Part model, mm, in its own coordinate system. Coordinates: 2 decimals unless noted, no trailing zeros. Loops run counter-clockwise (first coordinate to the right, second up) from the corner with the lowest first, then second, coordinate; pieces in that order, holes last. Notation, with made-up numbers: (-25.5, 3.25) - (-4.5, 3.25) arc R12 cw to (-4.5, 14.25) - close; hole circle Ø4 at (-8.75, 41.5). An arc over 180 degrees is marked (long way). Use a Markdown table: item, result. Add a question column.
1. Band-saw the part on A-A, the plane y = 133.5. Give the cut face in (x, z).
2. Wall check: probe 1 along Y at (x, z) = (48.8, 3.4); probe 2 along X at (y, z) = (133.5, 3.25); probe 3 along X at (y, z) = (41.5, 1.8). Give the ranges that are in metal, low to high. Write a range as [from, to].
3. Band-saw the part on C-C, the plane x = 28.8. Give the cut face in (y, z), plus the area to 3 significant figures.
4. Band-saw the part on B-B, the plane z = 3.85. Count the separate pieces of the cut face and the enclosed holes in it, plus the area to 3 significant figures.
5. Drop flat-ended pins along their axis: pin 1 (2 mm diameter, centred on y = 82, z = 2.5, fed in from +X); pin 2 (1.5 mm diameter, centred on y = 3.5, z = 1.5, fed in from +X); pin 3 (1.5 mm diameter, centred on x = 3.5, z = 1.5, fed in from +Y). Give the stop position or say it passes through.
6. Band-saw the part on D-D, the plane y = 75.5. Give the cut face in (x, z), plus the area to 3 significant figures.
from build123d import *

# Parameters (mm, degrees)
SKETCH_1_W          = 77.6
SKETCH_1_H          = 137
EXTRUDE_1_DEPTH     = 5
SKETCH_3_W          = 18.8
SKETCH_3_H          = 7.5
SKETCH_3_W_2        = 5
SKETCH_3_H_2        = 30
CUT_EXTRUDE_1_DEPTH = 5
SKETCH_4_R          = 2
CUT_EXTRUDE_2_DEPTH = 5
SKETCH_5_W          = 55
SKETCH_5_H          = 110
CUT_EXTRUDE_3_DEPTH = 7
FILLET_1_R          = 10
SKETCH_7_W          = 40
SKETCH_7_H          = 0.5
EXTRUDE_2_DEPTH     = 5


with BuildPart() as part:
    # 草图1 → 凸台-拉伸1 (new body)
    with BuildSketch(Plane.XY):
        with Locations((38.8, 68.5)):
            Rectangle(SKETCH_1_W, SKETCH_1_H)
    extrude(amount=EXTRUDE_1_DEPTH)

    # 草图3 → 切除-拉伸1 (cut)
    with BuildSketch(Plane.XY.offset(5)):
        with Locations((9.4, 133.25)):
            Rectangle(SKETCH_3_W, SKETCH_3_H)
        with Locations((9.4, 3.75)):
            Rectangle(SKETCH_3_W, SKETCH_3_H)
        with Locations((68.2, 3.75)):
            Rectangle(SKETCH_3_W, SKETCH_3_H)
        with Locations((68.2, 133.25)):
            Rectangle(SKETCH_3_W, SKETCH_3_H)
        with Locations((75.1, 68.5)):
            Rectangle(SKETCH_3_W_2, SKETCH_3_H_2)
        with Locations((2.5, 68.5)):
            Rectangle(SKETCH_3_W_2, SKETCH_3_H_2)
    extrude(amount=-CUT_EXTRUDE_1_DEPTH, mode=Mode.SUBTRACT)

    # 草图4 → 切除-拉伸2 (cut)
    with BuildSketch(Plane.XY.offset(5)):
        with Locations((28.8, 133.5)):
            Circle(SKETCH_4_R)
        with Locations((48.8, 133.5)):
            Circle(SKETCH_4_R)
        with Locations((28.8, 3.5)):
            Circle(SKETCH_4_R)
        with Locations((48.8, 3.5)):
            Circle(SKETCH_4_R)
    extrude(amount=-CUT_EXTRUDE_2_DEPTH, mode=Mode.SUBTRACT)

    # 草图5 → 切除-拉伸3 (cut)
    with BuildSketch(Plane(origin=(0, 0, 0), x_dir=(-1, 0, 0), z_dir=(0, 0, -1))):
        with Locations((-38.8, 68)):
            Rectangle(SKETCH_5_W, SKETCH_5_H)
    extrude(amount=-CUT_EXTRUDE_3_DEPTH, mode=Mode.SUBTRACT)

    # 圆角1
    fillet_1_edges = [part.edges().sort_by_distance(p)[0] for p in [
        (66.3, 13, 2.5),
        (66.3, 123, 2.5),
        (11.3, 123, 2.5),
        (11.3, 13, 2.5),
    ]]
    fillet(fillet_1_edges, radius=FILLET_1_R)

    # 草图7 → 凸台-拉伸2 (add)
    with BuildSketch(Plane.XY.offset(5)):
        with Locations((38.8, 137.25)):
            Rectangle(SKETCH_7_W, SKETCH_7_H)
        with Locations((38.8, -0.25)):
            Rectangle(SKETCH_7_W, SKETCH_7_H)
    extrude(amount=-EXTRUDE_2_DEPTH)


solid = part.part
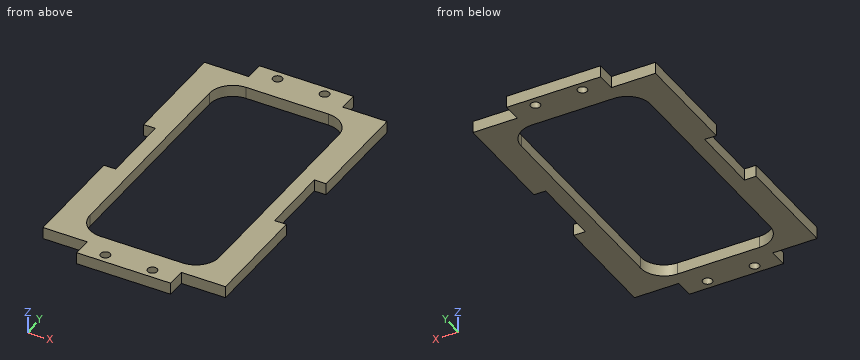
Geometry check:
| question | item | result |
|---|---|---|
| 1 | outline | (18.8, 0) - (26.8, 0) - (26.8, 5) - (18.8, 5) - close; (30.8, 0) - (46.8, 0) - (46.8, 5) - (30.8, 5) - close; (50.8, 0) - (58.8, 0) - (58.8, 5) - (50.8, 5) - close |
| 2 | probe 1 | y = [-0.5, 1.5], [5.5, 13], [123, 131.5], [135.5, 137.5] |
| 2 | probe 2 | x = [18.8, 26.8], [30.8, 46.8], [50.8, 58.8] |
| 2 | probe 3 | x = [0, 11.3], [66.3, 77.6] |
| 3 | outline | (-0.5, 0) - (1.5, 0) - (1.5, 5) - (-0.5, 5) - close; (5.5, 0) - (13, 0) - (13, 5) - (5.5, 5) - close; (123, 0) - (131.5, 0) - (131.5, 5) - (123, 5) - close; (135.5, 0) - (137.5, 0) - (137.5, 5) - (135.5, 5) - close |
| 3 | area | 100 mm^2 |
| 4 | separate pieces | 1 |
| 4 | enclosed holes | 5 |
| 4 | area | 3,790 mm^2 |
| 5 | pin 1 | stops at x = 72.6 |
| 5 | pin 2 | stops at x = 58.8 |
| 5 | pin 3 | stops at y = 129.5 |
| 6 | outline | (5, 0) - (11.3, 0) - (11.3, 5) - (5, 5) - close; (66.3, 0) - (72.6, 0) - (72.6, 5) - (66.3, 5) - close |
| 6 | area | 63.0 mm^2 |
